Design review of the part built by this model. Coordinates are the model's own, in mm. A direction names the side the tool comes from. Coordinates: 2 decimals unless noted, no trailing zeros. Order: outer loops, then holes, each group sorted by start corner. A loop starts at its lowest first (then second) coordinate and runs counter-clockwise, first axis right, second up. Notation, with made-up numbers: (32, 17) - (54, 17) arc R13 ccw to (54, 31) - close; hole circle Ø7 at (53, -12). An arc over 180 degrees is marked (long way). Write each question's results on one line, items separated by ' | '. Start each with the question number.
```python
from build123d import *

# Parameters (mm, degrees)
CLOSED_BOTTOM_PLATE_3MM_DEPTH   = 3
FOOT1_CURVED_R70P71_DEPTH       = 20
FOOT2_CURVED_R70P71_DEPTH       = 20
PAD4_C_BLANK_DEPTH              = 20
PAD5_A_BLANK_DEPTH              = 20
SLOT_BACKING_INSIDE_NORTH_DEPTH = 22
SLOT_BACKING_INSIDE_EAST_DEPTH  = 22
TOP_OUTER_PLANE_DEPTH           = 157.633329786
TOP_OUTER_PLANE_DEPTH_BACK      = 157.633329786
SLOT_BASE_NORTH_DEPTH           = 3
SLOT_BASE_EAST_DEPTH            = 3
SLOT_OUTER_NORTH_DEPTH          = 22
SLOT_OUTER_EAST_DEPTH           = 22
CUT_EXTRUDE_2_DEPTH             = 165.335023656
CUT_EXTRUDE_2_DEPTH_BACK        = 165.335023656


with BuildPart() as part:
    # Closed_bottom_plate_3mm_sketch → Closed_bottom_plate_3mm (new body)
    with BuildSketch(Plane.XY):
        with BuildLine():
            Line((77.781745931, -63.639610307), (141.421356237, 0))
            Line((141.421356237, 0), (77.781745931, 63.639610307))
            Line((77.781745931, 63.639610307), (56.568542495, 42.426406871))
            ThreePointArc((56.568542495, 42.426406871), (70.710678119, 0), (56.568542495, -42.426406871))
            Line((56.568542495, -42.426406871), (77.781745931, -63.639610307))
        make_face()
    extrude(amount=CLOSED_BOTTOM_PLATE_3MM_DEPTH)

    # Foot1_curved_R70p71_sketch → Foot1_curved_R70p71 (add)
    with BuildSketch(Plane.XY):
        with BuildLine():
            Line((62.225396744, 48.083261121), (67.882250994, 42.426406871))
            Line((67.882250994, 42.426406871), (61.080791676, 35.624947554))
            ThreePointArc((61.080791676, 35.624947554), (58.922885367, 39.090837546), (56.568542495, 42.426406871))
            Line((56.568542495, 42.426406871), (62.225396744, 48.083261121))
        make_face()
    extrude(amount=FOOT1_CURVED_R70P71_DEPTH)

    # Foot2_curved_R70p71_sketch → Foot2_curved_R70p71 (add)
    with BuildSketch(Plane.XY):
        with BuildLine():
            Line((62.225396744, -48.083261121), (67.882250994, -42.426406871))
            Line((67.882250994, -42.426406871), (61.080791676, -35.624947554))
            ThreePointArc((61.080791676, -35.624947554), (58.922885367, -39.090837546), (56.568542495, -42.426406871))
            Line((56.568542495, -42.426406871), (62.225396744, -48.083261121))
        make_face()
    extrude(amount=FOOT2_CURVED_R70P71_DEPTH)

    # Pad4_C_blank_sketch → Pad4_C_blank (add)
    with BuildSketch(Plane.XY):
        Polygon((72.124891681, 57.982756057), (77.781745931, 52.325901808), (83.43860018, 57.982756057), (77.781745931, 63.639610307), align=None)
    extrude(amount=PAD4_C_BLANK_DEPTH)

    # Pad5_A_blank_sketch → Pad5_A_blank (add)
    with BuildSketch(Plane.XY):
        Polygon((72.124891681, -57.982756057), (77.781745931, -63.639610307), (83.43860018, -57.982756057), (77.781745931, -52.325901808), align=None)
    extrude(amount=PAD5_A_BLANK_DEPTH)

    # Slot_backing_inside_north_sketch → Slot_backing_inside_north (add)
    with BuildSketch(Plane.XY):
        Polygon((117.379725677, 18.384776311), (138.592929113, -2.828427125), (141.421356237, 0), (120.208152802, 21.213203436), align=None)
    extrude(amount=SLOT_BACKING_INSIDE_NORTH_DEPTH)

    # Slot_backing_inside_east_sketch → Slot_backing_inside_east (add)
    with BuildSketch(Plane.XY):
        Polygon((117.379725677, -18.384776311), (120.208152802, -21.213203436), (141.421356237, 0), (138.592929113, 2.828427125), align=None)
    extrude(amount=SLOT_BACKING_INSIDE_EAST_DEPTH)

    # Top_outer_plane_sketch → Top_outer_plane (cut, two sides: drawn at the far end of the back side and taken through both)
    with BuildSketch(Plane(origin=(0, 0, 0), x_dir=(1, 0, 0), z_dir=(0, 1, 0)).offset(-TOP_OUTER_PLANE_DEPTH_BACK)):
        Polygon((-100, 24.67766953), (250, -37.194173824), (250, -100), (-100, -100), align=None)
    extrude(amount=TOP_OUTER_PLANE_DEPTH + TOP_OUTER_PLANE_DEPTH_BACK, mode=Mode.SUBTRACT)

    # Slot_base_north_sketch → Slot_base_north (add)
    with BuildSketch(Plane.XY):
        Polygon((117.379725677, 18.384776311), (142.8355698, -7.071067812), (149.906637612, 0), (124.450793489, 25.455844123), align=None)
    extrude(amount=SLOT_BASE_NORTH_DEPTH)

    # Slot_base_east_sketch → Slot_base_east (add)
    with BuildSketch(Plane.XY):
        Polygon((117.379725677, -18.384776311), (124.450793489, -25.455844123), (149.906637612, 0), (142.8355698, 7.071067812), align=None)
    extrude(amount=SLOT_BASE_EAST_DEPTH)

    # Slot_outer_north_sketch → Slot_outer_north (add)
    with BuildSketch(Plane.XY):
        Polygon((122.329473145, 23.334523779), (147.785317268, -2.121320344), (149.906637612, 0), (124.450793489, 25.455844123), align=None)
    extrude(amount=SLOT_OUTER_NORTH_DEPTH)

    # Slot_outer_east_sketch → Slot_outer_east (add)
    with BuildSketch(Plane.XY):
        Polygon((122.329473145, -23.334523779), (124.450793489, -25.455844123), (149.906637612, 0), (147.785317268, 2.121320344), align=None)
    extrude(amount=SLOT_OUTER_EAST_DEPTH)

    # 草图13 → 切除-拉伸2 (cut, two sides: drawn at the far end of the back side and taken through both)
    with BuildSketch(Plane(origin=(0, 0, 0), x_dir=(1, 0, 0), z_dir=(0, 1, 0)).offset(-CUT_EXTRUDE_2_DEPTH_BACK)):
        Polygon((-100, 22.646659929), (250, -39.225183425), (250, -100), (-100, -100), align=None)
    extrude(amount=CUT_EXTRUDE_2_DEPTH + CUT_EXTRUDE_2_DEPTH_BACK, mode=Mode.SUBTRACT)


solid = part.part
```
(1) Take a section at A-A (x = 130.5). State the section outline as (y, z) points, plus the area to 3 significant figures.
(2) Take a section at B-B (y = 9). State the section outline as (x, z) points.
(3) Clearance check with flat-ended pins moving along their axes: pin 1 (12.5 mm diameter, centred on x = 128, y = -5.5, fed in from +Z); pin 2 (3 mm diameter, centred on x = 86, y = -50.5, fed in from +Z); pin 3 (8 mm diameter, centred on y = -6, z = 10.5, fed in from +X). State where each tip first meets the part, or that it passes through.
(4) Take a section at C-C (z = 1.5). State the section outline as (x, y) points.
(5) Mouldability with a two-part tool opening along X and no side actions: class faces 1 (the face through (137.357, 12.55, 10.615)), 2 (the face through (140.139, -5.776, 19.804)), 3 (the face through (123.243, -24.248, 6.504)) as +X half, -X half, draft (parallel to the pull), parting line (faces both ways), or undercut.
(6) To check wall thickness, follow line 1 along Z through (x, y) = (75.5, 0); line 2 along Y through (x, z) = (117.5, 8.75); line 3 along Z through (x, y) = (145.5, 4). State the ranges of each line that lie inside material, in increasing order. Write a range as [from, to].
(7) Tool access review of faces 4 (the face through (126.443, 9.321, 9.902)), 5 (the face through (65.014, 45.294, 3.764)), 6 (the face through (118.814, 19.819, 8.546)): name each direction out of +Z, -Z, +X, -X, +Y, -Y from which nothing blocks a thin tool from reaching the whole face with its end or side.
(8) Take a section at D-D (x = 66.5). State the section outline as (y, z) points.
Worked out:
1) outline: (-19.41, 0) - (19.41, 0) - (19.41, 18.1) - (15.16, 18.1) - (15.16, 3) - (10.92, 3) - (10.92, 16.07) - (5.26, 16.07) - (5.26, 3) - (-5.26, 3) - (-5.26, 16.07) - (-10.92, 16.07) - (-10.92, 3) - (-15.16, 3) - (-15.16, 18.1) - (-19.41, 18.1) - close | area: 392 mm^2
2) outline: (70.14, 0) - (140.91, 0) - (140.91, 19.94) - (136.66, 19.19) - (136.66, 3) - (132.42, 3) - (132.42, 16.41) - (126.76, 15.41) - (126.76, 3) - (70.14, 3) - close
3) pin 1: z = 16.73 | pin 2: z = 3 | pin 3: x = 147.91
4) outline: (56.57, -42.43) - (77.78, -63.64) - (120.21, -21.21) - (124.45, -25.46) - (149.91, 0) - (124.45, 25.46) - (120.21, 21.21) - (77.78, 63.64) - (56.57, 42.43) arc R70.71 cw to start
5) face 1: +X half | face 2: -X half | face 3: undercut
6) line 1: [0, 3] | line 2: [-18.51, -18.26], [18.26, 18.51] | line 3: [0, 20.75]
7) face 4: +Z, -X | face 5: +Z, +X, +Y | face 6: +Z, -X, +Y
8) outline: (-52.36, 0) - (-24.04, 0) - (-24.04, 3) - (-41.04, 3) - (-41.04, 4.76) - (-43.81, 4.76) - (-43.81, 3) - (-52.36, 3) - close; (24.04, 0) - (52.36, 0) - (52.36, 3) - (43.81, 3) - (43.81, 4.76) - (41.04, 4.76) - (41.04, 3) - (24.04, 3) - close
